```python
from build123d import *

# Parameters (mm, degrees)
SZKIC1_W                    = 25
SZKIC1_H                    = 44.2
DODANIE_WYCI_GNI_CIE1_DEPTH = 3
ZAOKR_GLENIE1_R             = 4.8
SZKIC2_R                    = 1.75
WYTNIJ_WYCI_GNI_CIE1_DEPTH  = 3
SFAZOWANIE1_SIZE            = 1


with BuildPart() as part:
    # Szkic1 → Dodanie-wyciągnięcie1 (new body)
    with BuildSketch(Plane.XY):
        Rectangle(SZKIC1_W, SZKIC1_H)
    extrude(amount=DODANIE_WYCI_GNI_CIE1_DEPTH)

    # Zaokrąglenie1
    zaokr_glenie1_edges = [part.edges().sort_by_distance(p)[0] for p in [
        (-12.5, 22.1, 1.5),
        (12.5, 22.1, 1.5),
        (12.5, -22.1, 1.5),
        (-12.5, -22.1, 1.5),
    ]]
    fillet(zaokr_glenie1_edges, radius=ZAOKR_GLENIE1_R)

    # Szkic2 → Wytnij-wyciągnięcie1 (cut)
    with BuildSketch(Plane.XY.offset(3)):
        with Locations((-8.7, -18.3)):
            Circle(SZKIC2_R)
        with Locations((8.7, -18.3)):
            Circle(SZKIC2_R)
        with BuildLine():
            Line((12.5, 11.95), (12.5, 15.45))
            Line((12.5, 15.45), (10.7, 15.45))
            ThreePointArc((10.7, 15.45), (11.937436867, 14.937436867), (12.45, 13.7))
            ThreePointArc((12.45, 13.7), (11.937436867, 12.462563133), (10.7, 11.95))
            Line((10.7, 11.95), (12.5, 11.95))
        make_face()
        with Locations((10.7, 13.7)):
            Circle(SZKIC2_R)
        with Locations((-10.7, 13.7)):
            Circle(SZKIC2_R)
        with BuildLine():
            ThreePointArc((-10.7, 11.95), (-12.45, 13.7), (-10.7, 15.45))
            Line((-10.7, 15.45), (-12.5, 15.45))
            Line((-12.5, 15.45), (-12.5, 11.95))
            Line((-12.5, 11.95), (-10.7, 11.95))
        make_face()
    extrude(amount=-WYTNIJ_WYCI_GNI_CIE1_DEPTH, mode=Mode.SUBTRACT)

    # Sfazowanie1
    sfazowanie1_edges = [part.edges().sort_by_distance(p)[0] for p in [
        (-11.6, 11.95, 3),
        (-8.95, 13.7, 3),
        (-11.6, 15.45, 3),
        (11.6, 11.95, 3),
        (11.6, 15.45, 3),
        (8.95, 13.7, 3),
        (6.95, -18.3, 3),
        (-10.45, -18.3, 3),
    ]]
    chamfer(sfazowanie1_edges, length=SFAZOWANIE1_SIZE)


solid = part.part
```
Input: part model. Units: mm. Frame: model coordinates. A direction names the side the tool comes from. Round coordinates to 2 decimals unless told otherwise and drop trailing zeros. Loops run counter-clockwise (first coordinate to the right, second up) from the corner with the lowest first, then second, coordinate; pieces in that order, holes last. Notation, with made-up numbers: (-27, 14) -> (-12, 14) arc R28 cw to (-12, 50) -> close; hole circle Ø5 at (-19.5, -13). An arc over 180 degrees is marked (long way). One line per item, written item: value.
(1) Section B-B (z = 0.8). Return the cut outline in (x, y), plus the area to 3 significant figures.
Geometry check:
outline: (-12.5, -17.3) arc R4.8 ccw to (-7.7, -22.1) -> (7.7, -22.1) arc R4.8 ccw to (12.5, -17.3) -> (12.5, 11.95) -> (10.7, 11.95) arc R1.75 cw to (10.7, 15.45) -> (12.5, 15.45) -> (12.5, 17.3) arc R4.8 ccw to (7.7, 22.1) -> (-7.7, 22.1) arc R4.8 ccw to (-12.5, 17.3) -> (-12.5, 15.45) -> (-10.7, 15.45) arc R1.75 cw to (-10.7, 11.95) -> (-12.5, 11.95) -> close; hole circle Ø3.5 at (-8.7, -18.3); hole circle Ø3.5 at (8.7, -18.3)
area: 1,040 mm2
(2) Material intervals for line 1 (Y direction, x = 10, z = 2.5); line 2 (Y direction, x = -11, z = 0.7); line 3 (Y direction, x = -8.7, z = 1.45), sorted ascending. Write a range as [from, to].
Geometry check:
line 1: [-21.51, -20.14], [-16.46, 11.56], [15.84, 21.51]
line 2: [-20.79, 11.95], [15.45, 20.79]
line 3: [-21.99, -20.05], [-16.55, 21.99]
(3) Section A-A (y = 13.7). Return the cut outline in (x, z), plus the area to 3 significant figures.
Geometry check:
outline: (-8.95, 0) -> (8.95, 0) -> (8.95, 2) -> (7.95, 3) -> (-7.95, 3) -> (-8.95, 2) -> close
area: 52.7 mm2
(4) Section C-C (y = -18.3). Return the cut outline in (x, z), plus the area to 3 significant figures.
Geometry check:
outline: (-12.39, 0) -> (-10.45, 0) -> (-10.45, 2) -> (-11.45, 3) -> (-12.39, 3) -> close; (-6.95, 0) -> (6.95, 0) -> (6.95, 2) -> (5.95, 3) -> (-5.95, 3) -> (-6.95, 2) -> close; (10.45, 0) -> (12.39, 0) -> (12.39, 3) -> (11.45, 3) -> (10.45, 2) -> close
area: 51.4 mm2
(5) Mould query, pull axis Y, two halves, no side actions, for faces 1 (the face through (11.59, 11.46, 2.49)), 2 (the face through (11.13, 20.66, 1.52)), 3 (the face through (0, 0, 0)). Classes: pulls with the +Y half, pulls with the -Y half, needs draft (parallel to the pull), parting line crosses it, or undercut.
Geometry check:
face 1: undercut
face 2: pulls with the +Y half
face 3: needs draft
(6) Set-up query: faces 4 (the face through (-11.61, 11.44, 2.51)), 5 (the face through (12, 11.95, 1)), 6 (the face through (-12.5, -3, 1)). Return all of +Z, -Z, +X, -X, +Y, -Y with unobstructed straight access to the full face (end or side cutting, diameter ignored); none if empty.
Geometry check:
face 4: +Z, -X
face 5: +Z, -Z, +X
face 6: +Z, -Z, -X, +Y, -Y
(7) Pin query (flat end, axial travel): pin 1 (0.9 mm diameter, centred on x = -11.5, z = 1, fed in from +Y); pin 2 (0.5 mm diameter, centred on x = 12, z = 0.5, fed in from -Y); pin 3 (2 mm diameter, centred on x = 8.7, y = -18.3, fed in from +Z). Return the tip coordinate at first contact, or that it passes through.
Geometry check:
pin 1: y = 20.74
pin 2: y = -19.88
pin 3: through
